Here's how the part is built. I have some questions about the finished solid (model axes, mm). Face numbers are marked on the shaded views. Give positions to 0.01 mm unless a question says otherwise; leave off trailing zeros. Loops run counter-clockwise (first coordinate to the right, second up) from the corner with the lowest first, then second, coordinate; pieces in that order, holes last. Notation, with made-up numbers: M 61,42 L 106,42 A24 ccw 106,76 Z; hole C -23,83 d10. An arc over 180 degrees is marked long. Write item = value, one per line. Start each with the question number.
```python
from build123d import *

# Parameters (mm, degrees)
F1_W     = 5
F1_H     = 2.5
F1_W_2   = 2.5
F1_H_2   = 5
F2_DEPTH = 15
F5_R     = 5


with BuildPart() as f2:
    # F1 (on Top) → F2 (new body)
    with BuildSketch(Plane.XY):
        with BuildLine():
            ThreePointArc((-26.0240273593, 5), (-18.7383297014, 18.7383297014), (-5, 26.0240273593))
            Line((-5, 26.0240273593), (-5, 29.5803989155))
            ThreePointArc((-5, 29.5803989155), (-21.2132034356, 21.2132034356), (-29.5803989155, 5))
            Line((-29.5803989155, 5), (-26.0240273593, 5))
        make_face()
        with BuildLine():
            ThreePointArc((-26.0240273593, -5), (-26.5, 0), (-26.0240273593, 5))
            Line((-26.0240273593, 5), (-29.5803989155, 5))
            ThreePointArc((-29.5803989155, 5), (-30, 0), (-29.5803989155, -5))
            Line((-29.5803989155, -5), (-26.0240273593, -5))
        make_face()
        with BuildLine():
            Line((-5, -29.5803989155), (-5, -26.0240273593))
            ThreePointArc((-5, -26.0240273593), (-18.7383297014, -18.7383297014), (-26.0240273593, -5))
            Line((-26.0240273593, -5), (-29.5803989155, -5))
            ThreePointArc((-29.5803989155, -5), (-21.2132034356, -21.2132034356), (-5, -29.5803989155))
        make_face()
        with BuildLine():
            Line((-24, 2.5), (-10, 2.5))
            Line((-10, 2.5), (-10, 5))
            Line((-10, 5), (-26.0240273593, 5))
            ThreePointArc((-26.0240273593, 5), (-26.5, 0), (-26.0240273593, -5))
            Line((-26.0240273593, -5), (-10, -5))
            Line((-10, -5), (-10, -2.5))
            Line((-10, -2.5), (-24, -2.5))
            Line((-24, -2.5), (-24, 2.5))
        make_face()
        with BuildLine():
            Line((5, -10), (2.5, -10))
            Line((2.5, -10), (2.5, -24))
            Line((2.5, -24), (-2.5, -24))
            Line((-2.5, -24), (-2.5, -10))
            Line((-2.5, -10), (-5, -10))
            Line((-5, -10), (-5, -26.0240273593))
            ThreePointArc((-5, -26.0240273593), (0, -26.5), (5, -26.0240273593))
            Line((5, -26.0240273593), (5, -10))
        make_face()
        with BuildLine():
            Line((10, 5), (10, 2.5))
            Line((10, 2.5), (24, 2.5))
            Line((24, 2.5), (24, -2.5))
            Line((24, -2.5), (10, -2.5))
            Line((10, -2.5), (10, -5))
            Line((10, -5), (26.0240273593, -5))
            ThreePointArc((26.0240273593, -5), (26.3807384755, -2.5113019509), (26.5, 0))
            ThreePointArc((26.5, 0), (26.3807384755, 2.5113019509), (26.0240273593, 5))
            Line((26.0240273593, 5), (10, 5))
        make_face()
        with BuildLine():
            Line((2.5, 24), (2.5, 10))
            Line((2.5, 10), (5, 10))
            Line((5, 10), (5, 26.0240273593))
            ThreePointArc((5, 26.0240273593), (0, 26.5), (-5, 26.0240273593))
            Line((-5, 26.0240273593), (-5, 10))
            Line((-5, 10), (-2.5, 10))
            Line((-2.5, 10), (-2.5, 24))
            Line((-2.5, 24), (2.5, 24))
        make_face()
        with BuildLine():
            Line((5, 29.5803989155), (5, 26.0240273593))
            ThreePointArc((5, 26.0240273593), (18.7383297014, 18.7383297014), (26.0240273593, 5))
            Line((26.0240273593, 5), (29.5803989155, 5))
            ThreePointArc((29.5803989155, 5), (21.2132034356, 21.2132034356), (5, 29.5803989155))
        make_face()
        with BuildLine():
            ThreePointArc((-5, 26.0240273593), (0, 26.5), (5, 26.0240273593))
            Line((5, 26.0240273593), (5, 29.5803989155))
            ThreePointArc((5, 29.5803989155), (0, 30), (-5, 29.5803989155))
            Line((-5, 29.5803989155), (-5, 26.0240273593))
        make_face()
        with BuildLine():
            Line((29.5803989155, 5), (26.0240273593, 5))
            ThreePointArc((26.0240273593, 5), (26.3807384755, 2.5113019509), (26.5, 0))
            ThreePointArc((26.5, 0), (26.3807384755, -2.5113019509), (26.0240273593, -5))
            Line((26.0240273593, -5), (29.5803989155, -5))
            ThreePointArc((29.5803989155, -5), (29.8949156836, -2.5087878084), (30, 0))
            ThreePointArc((30, 0), (29.8949156836, 2.5087878084), (29.5803989155, 5))
        make_face()
        with BuildLine():
            ThreePointArc((2.5, 3.4369317712), (3.00520382, 3.00520382), (3.4369317712, 2.5))
            Line((3.4369317712, 2.5), (5, 2.5))
            Line((5, 2.5), (5, 5))
            Line((5, 5), (2.5, 5))
            Line((2.5, 5), (2.5, 3.4369317712))
        make_face()
        with BuildLine():
            ThreePointArc((-2.5, 3.4369317712), (0, 4.25), (2.5, 3.4369317712))
            Line((2.5, 3.4369317712), (2.5, 5))
            Line((2.5, 5), (-2.5, 5))
            Line((-2.5, 5), (-2.5, 3.4369317712))
        make_face()
        with BuildLine():
            ThreePointArc((-3.4369317712, 2.5), (-3.00520382, 3.00520382), (-2.5, 3.4369317712))
            Line((-2.5, 3.4369317712), (-2.5, 5))
            Line((-2.5, 5), (-5, 5))
            Line((-5, 5), (-5, 2.5))
            Line((-5, 2.5), (-3.4369317712, 2.5))
        make_face()
        with BuildLine():
            ThreePointArc((-3.4369317712, -2.5), (-4.25, 0), (-3.4369317712, 2.5))
            Line((-3.4369317712, 2.5), (-5, 2.5))
            Line((-5, 2.5), (-5, -2.5))
            Line((-5, -2.5), (-3.4369317712, -2.5))
        make_face()
        with BuildLine():
            Line((-2.5, -5), (-2.5, -3.4369317712))
            ThreePointArc((-2.5, -3.4369317712), (-3.00520382, -3.00520382), (-3.4369317712, -2.5))
            Line((-3.4369317712, -2.5), (-5, -2.5))
            Line((-5, -2.5), (-5, -5))
            Line((-5, -5), (-2.5, -5))
        make_face()
        with BuildLine():
            Line((2.5, -5), (2.5, -3.4369317712))
            ThreePointArc((2.5, -3.4369317712), (0, -4.25), (-2.5, -3.4369317712))
            Line((-2.5, -3.4369317712), (-2.5, -5))
            Line((-2.5, -5), (2.5, -5))
        make_face()
        with BuildLine():
            Line((5, -2.5), (3.4369317712, -2.5))
            ThreePointArc((3.4369317712, -2.5), (3.00520382, -3.00520382), (2.5, -3.4369317712))
            Line((2.5, -3.4369317712), (2.5, -5))
            Line((2.5, -5), (5, -5))
            Line((5, -5), (5, -2.5))
        make_face()
        with BuildLine():
            ThreePointArc((3.4369317712, 2.5), (4.041624675, 1.3144466464), (4.25, 0))
            ThreePointArc((4.25, 0), (4.041624675, -1.3144466464), (3.4369317712, -2.5))
            Line((3.4369317712, -2.5), (5, -2.5))
            Line((5, -2.5), (5, 2.5))
            Line((5, 2.5), (3.4369317712, 2.5))
        make_face()
        with BuildLine():
            ThreePointArc((26.0240273593, -5), (18.7383297014, -18.7383297014), (5, -26.0240273593))
            Line((5, -26.0240273593), (5, -29.5803989155))
            ThreePointArc((5, -29.5803989155), (21.2132034356, -21.2132034356), (29.5803989155, -5))
            Line((29.5803989155, -5), (26.0240273593, -5))
        make_face()
        with BuildLine():
            Line((5, -29.5803989155), (5, -26.0240273593))
            ThreePointArc((5, -26.0240273593), (0, -26.5), (-5, -26.0240273593))
            Line((-5, -26.0240273593), (-5, -29.5803989155))
            ThreePointArc((-5, -29.5803989155), (0, -30), (5, -29.5803989155))
        make_face()
        with Locations((-7.5, 3.75)):
            Rectangle(F1_W, F1_H)
        with Locations((7.5, 3.75)):
            Rectangle(F1_W, F1_H)
        with Locations((3.75, -7.5)):
            Rectangle(F1_W_2, F1_H_2)
        with Locations((0, -7.5)):
            Rectangle(F1_W, F1_H_2)
        with Locations((-3.75, -7.5)):
            Rectangle(F1_W_2, F1_H_2)
        with Locations((-7.5, -3.75)):
            Rectangle(F1_W, F1_H)
        with Locations((7.5, -3.75)):
            Rectangle(F1_W, F1_H)
        with Locations((3.75, 7.5)):
            Rectangle(F1_W_2, F1_H_2)
        with Locations((0, 7.5)):
            Rectangle(F1_W, F1_H_2)
        with Locations((-7.5, 0)):
            Rectangle(F1_W, F1_H_2)
        with Locations((7.5, 0)):
            Rectangle(F1_W, F1_H_2)
        with Locations((-3.75, 7.5)):
            Rectangle(F1_W_2, F1_H_2)
    extrude(amount=F2_DEPTH)

    # F3 (on Front) → F4 (revolve, cut)
    with BuildSketch(Plane.XZ):
        Polygon((-30, 15), (-30, 2.7), (-15, 15), align=None)
    revolve(axis=Axis((0, 0, 7.5), (0, 0, 1)), mode=Mode.SUBTRACT)

    # F5
    f5_edges = [f2.edges().sort_by_distance(p)[0] for p in [
        (5, 5, 7.5),
        (5, -5, 7.5),
        (-5, -5, 7.5),
        (-5, 5, 7.5),
    ]]
    fillet(f5_edges, radius=F5_R)


solid = f2.part
```
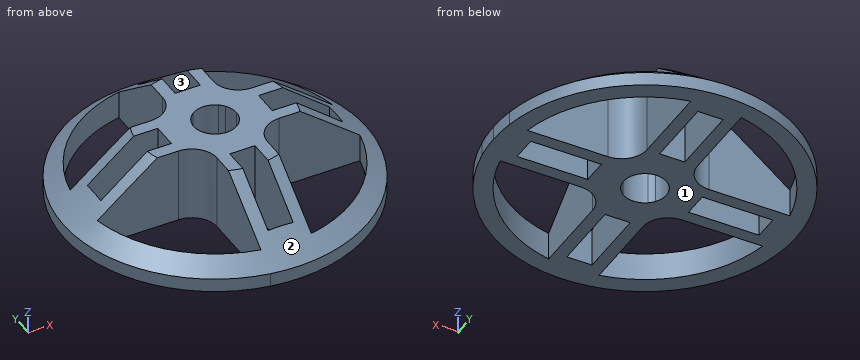
Q1. If I drill on line 1 along X through (y, z) = (14, 14.5); line 2 along X through (y, z) = (-12.5, 2.75), over which ranges is the centre line in solid material (lowest first)?
Q2. If we section it at A-A, the plane x = 0: List the corners of the cut face in (y, z) for me.
Q3. We'd pull the mould along X, two halves only. Please class the marked faces 1, 2 and 3: pulls with the +X half, pulls with the -X half, needs draft (parallel to the pull), parting line crosses it, or undercut.
Q4. Will these pins go through, and if not, where does the flat tip stop? pin 1 (2.5 mm diameter, centred on y = 0, z = 5.5, fed in from -X); pin 2 (6 mm diameter, centred on y = -18, z = 7, fed in from +X); pin 3 (1.5 mm diameter, centred on x = -6.5, z = 10, fed in from +Y).
Q5. If we section it at B-B, the plane z = 4.25: State how many separate pieces and enclosed holes the cut face has, then the cut area to 3 significant figures.
Resolved:
q1.line_1 = -5 to -2.5, 2.5 to 5
q1.line_2 = -27.2 to -23.37, -5 to -2.5, 2.5 to 5, 23.37 to 27.2
q2.outline = M -30,0 L -24,0 L -24,7.62 L -30,2.7 Z; M -10,0 L -4.25,0 L -4.25,15 L -10,15 Z; M 4.25,0 L 10,0 L 10,15 L 4.25,15 Z; M 24,0 L 30,0 L 30,2.7 L 24,7.62 Z
q3.face_1 = needs draft
q3.face_2 = parting line crosses it
q3.face_3 = undercut
q4.pin_1 = -28.11
q4.pin_2 = 22.54
q4.pin_3 = 7.37
q5.separate_pieces = 1
q5.enclosed_holes = 9
q5.area = 915 mm²
